Autodesk Inventor part; units mm, degrees
ref_plane "YZ Plane" through (0, 0, 0) normal (1, 0, 0) x (0, 1, 0)
ref_plane "XZ Plane" through (0, 0, 0) normal (0, 1, 0) x (-1, 0, 0)
ref_plane "XY Plane" through (0, 0, 0) normal (0, 0, 1) x (1, 0, 0)
sketch "Sketch1" plane through (0, 0, 0) normal (0, 0, 1) x (1, 0, 0)
  line L0 (-38, 45.376) -> (-29, 45.376)
  line L1 (-29, 45.376) -> (-29, 48)
  line L2 (-29, 141) -> (-29, 48)
  line L3 (-38, 141) -> (-29, 141)
  line L4 (-38, 45.376) -> (-38, 141)
  line L5 (0, 45.376) -> (45, 45.376)
  line L6 (45, 138) -> (45, 45.376)
  line L7 (33, 138) -> (45, 138)
  line L8 (33, 48) -> (33, 138)
  line L9 (6, 48) -> (33, 48)
  line L10 (6, 48) -> (6, 123)
  line L11 (6, 123) -> (-8.5, 123)
  line L12 (-8.5, 123) -> (-8.5, 48)
  line L13 (0, 48) -> (-8.5, 48)
  line L14 (0, 45.376) -> (0, 48)
  line L15 (0, 48) -> (0, 45.376)
  line L16 (-29, 48) -> (0, 48)
  line L17 (-29, 45.376) -> (-29, 48)
  line L18 (0, 45.376) -> (-29, 45.376)
  point P0 (0, 0)
  point P1 (276, 309.9765)
  dimension "GRIP3_W" = 12
  dimension "GRIP3_MID_THICK" = 14.5
  dimension "GRIP3_LEFT_THICK" = 9
  dimension "GRIP3_H" = 92.624
  dimension "GRIP3_MIDDLE_H" = 75
  dimension "GRIP3_LEFT_H" = 95.624
  dimension "GRIP3_W_ALL" = 83
  dimension "GRIP3_T" = 2.624
  dimension "GRIP3_T_2" = 2.624
extrude "Extrusion1" add sketch "Sketch1" along normal mid plane 70
sketch "Sketch2" plane through (0, 0, 0) normal (0, 0, 1) x (1, 0, 0)
  line L0 (-29, 45.376) -> (45, 45.376)
  line L1 (-15, 45.376) -> (-10, 45.376)
  line L2 (-10, 45.376) -> (-10, -24.624)
  line L3 (-10, -24.624) -> (-15, -24.624)
  line L4 (-15, -24.624) -> (-15, 45.376)
  line L5 (17, 45.376) -> (22, 45.376)
  line L6 (22, 45.376) -> (22, -24.624)
  line L7 (22, -24.624) -> (17, -24.624)
  line L8 (17, -24.624) -> (17, 45.376)
  line L9 (45, 45.376) -> (45, 138)
  line L10 (-38, 141) -> (-38, 45.376)
  point P0 (0, 0)
  point P1 (-10, 45.376)
  point P2 (22, 45.376)
  dimension "GRIP3_MTG" = 70
  dimension "GRIP3_MTG_TH" = 5
  dimension "GRIP3_LOC" = 23
  dimension "d16" = 23
extrude "Extrusion2" add sketch "Sketch2" along normal mid plane 35
sketch "Sketch3" plane through (0, 0, 0) normal (1, 0, 0) x (0, 1, 0)
  circle A0 centre (-16.624, 0) radius 4.123
  line L0 (-24.624, -17.5) -> (-24.624, 17.5)
  line L1 (45.376, -17.5) -> (-24.624, -17.5)
  point P0 (0, 0)
  dimension "PIN_HOLE_DIAM" = 8.246
  dimension "LOC_PIN_HOLE" = 8
  dimension "LOC_HOLE" = 17.5
extrude "Extrusion3" cut sketch "Sketch3" along normal blind 35 and the other way blind 35
sketch "Sketch4" plane through (45, 45.376, 35) normal (1, 0, 0) x (0, 0, -1)
  circle A0 centre (35, 46.312) radius 10
  line L0 (70, 92.624) -> (70, 0)
  line L1 (70, 0) -> (0, 0)
  point P0 (35, -45.376)
  dimension "PIN_DIAM1" = 20
  dimension "LOC_PIN" = 35
  dimension "d26" = 46.312
extrude "Extrusion4" add sketch "Sketch4" along normal blind 19.946
sketch "Sketch5" plane through (64.946, 91.688, 0) normal (1, 0, 0) x (0, 0, -1)
  circle A0 centre (0, 0) radius 7
  point P0 (0, -91.688)
  dimension "PIN_DIAME2" = 14
extrude "Extrusion5" add sketch "Sketch5" along normal blind 20
sketch "Sketch6" plane through (84.946, 91.688, 0) normal (1, 0, 0) x (0, 0, -1)
  circle A0 centre (0, 0) radius 10
  point P0 (0, -91.688)
  dimension "PIN_DIAM3" = 20
extrude "Extrusion6" add sketch "Sketch6" along normal blind 14
equation "\"GRIP3_T_2\" = GRIP3_T"
equation "\"d16\" = GRIP3_LOC"
equation "\"LOC_HOLE\" = 0.5 * GRIP3_MTG_EXTR"
equation "\"LOC_PIN\" = 0.5 * GRIP3_EXTR"
equation "\"d26\" = 0.5 * GRIP3_H"
equation "\"PIN_DIAM3\" = PIN_DIAM1"
equation "\"PIN3_H\" = PIN_DIAME2"
properties part number "grip - Copy1-1"
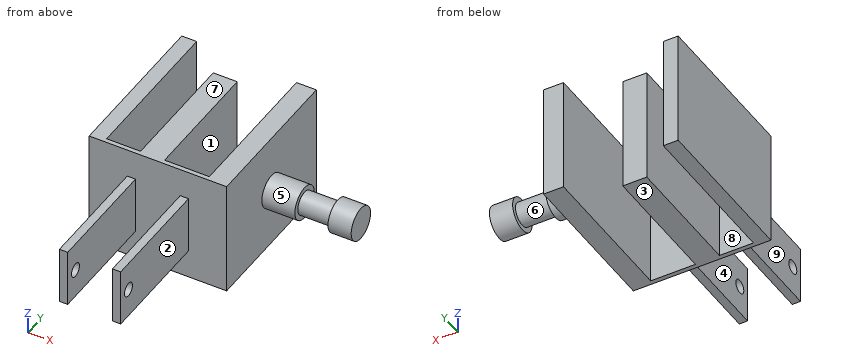
Work out the finished part from the listing and answer in its coordinate system (mm). Face numbers are marked on the shaded views. A direction names the side the tool comes from. Give positions to 0.01 mm unless a question says otherwise; leave off trailing zeros. Loops run counter-clockwise (first coordinate to the right, second up) from the corner with the lowest first, then second, coordinate; pieces in that order, holes last. Notation, with made-up numbers: (41, -0.5) -> (70, -0.5) arc R9 ccw to (70, 4.5) -> close; hole circle Ø11 at (40, -21). An arc over 180 degrees is marked (long way). Use a Markdown table: item, result. Add a question column.
1. Section A-A on y = 64 is taken. Determine the outline of the cut face in (x, z), and give its area (4 significant figures).
2. Flat-ended cylindrical pins translate along their axes: pin 1 Ø2.5 at (x, y) = (-13.5, 26) entering from -Z; pin 2 Ø10.5 at (y, z) = (16, 8) entering from -X; pin 3 Ø12 at (x, z) = (35.5, -0.5) entering from -Y. Find the tip coordinate at first contact, or state that the pin passes through.
3. Section C-C on z = 24 is taken. Determine the outline of the cut face in (x, y).
4. Section B-B on y = 37.5 is taken. Determine the outline of the cut face in (x, z), and give its area (3 significant figures).
5. Find the intervals of material crossed by probe 1 along X at (y, z) = (79.5, -15); probe 2 along X at (y, z) = (-2, 6); probe 3 along Y at (x, z) = (19.05, 0), in increasing order.
6. Section D-D on x = 14 is taken. Determine the outline of the cut face in (y, z), and give its area (3 significant figures).
7. Determine the mould class of the marked faces 1, 2, 3 and 4 for opening direction X: released by +X, released by -X, zero draft, split by the parting line, or undercut.
8. For the marked faces 5, 6, 7, 8 and 9, determine the directions among +Z, -Z, +X, -X, +Y, -Y from which every point of the face is accessible in a straight line to the end or side of a thin tool.
Results below:
| question | item | result |
|---|---|---|
| 1 | outline | (-38, -35) -> (-29, -35) -> (-29, 35) -> (-38, 35) -> close; (-8.5, -35) -> (6, -35) -> (6, 35) -> (-8.5, 35) -> close; (33, -35) -> (45, -35) -> (45, 35) -> (33, 35) -> close |
| 1 | area | 2,485 mm^2 |
| 2 | pin 1 | stops at z = -17.5 |
| 2 | pin 2 | stops at x = -15 |
| 2 | pin 3 | stops at y = 45.38 |
| 3 | outline | (-38, 45.38) -> (45, 45.38) -> (45, 138) -> (33, 138) -> (33, 48) -> (6, 48) -> (6, 123) -> (-8.5, 123) -> (-8.5, 48) -> (-29, 48) -> (-29, 141) -> (-38, 141) -> close |
| 4 | outline | (-15, -17.5) -> (-10, -17.5) -> (-10, 17.5) -> (-15, 17.5) -> close; (17, -17.5) -> (22, -17.5) -> (22, 17.5) -> (17, 17.5) -> close |
| 4 | area | 350 mm^2 |
| 5 | probe 1 | x = -38 to -29, -8.5 to 6, 33 to 45 |
| 5 | probe 2 | x = -15 to -10, 17 to 22 |
| 5 | probe 3 | y = -24.62 to -20.75, -12.5 to 48 |
| 6 | outline | (45.38, -35) -> (48, -35) -> (48, 35) -> (45.38, 35) -> close |
| 6 | area | 184 mm^2 |
| 7 | face 1 | undercut |
| 7 | face 2 | released by +X |
| 7 | face 3 | zero draft |
| 7 | face 4 | undercut |
| 8 | face 5 | +X |
| 8 | face 6 | none |
| 8 | face 7 | +Z, +X, -X, +Y, -Y |
| 8 | face 8 | +Z, -Z, +Y |
| 8 | face 9 | +Z, -Z, -X, -Y |
